For this review, take the finished solid that the model builds, in its own axes (mm). A direction names the side the tool comes from. Give positions to 0.01 mm unless a question says otherwise; leave off trailing zeros. Write each loop counter-clockwise with the first axis right and the second up, starting at its lowest first coordinate (ties: lowest second). Pieces come first, ordered by that corner, then holes. Notation, with made-up numbers: M -16.5,54.5 L -3.5,54.5 A20 ccw -3.5,87.5 Z; hole C 59,0.25 d9. An arc over 180 degrees is marked long. Write item = value, one per line.
```python
from build123d import *

# Parameters (mm, degrees)
SKETCH1_W           = 45
SKETCH1_H           = 6
BOSS_EXTRUDE1_DEPTH = 6


with BuildPart() as part:
    # Sketch1 → Boss-Extrude1 (new body)
    with BuildSketch(Plane.XY):
        Polygon((127.972610893, -160.108528092), (-86.474936563, -160.108528092), (-86.474936563, -401.007755411), (127.972610893, -401.007755411), (157.972610893, -401.007755411), (163.972610893, -401.007755411), (163.972610893, -366.007755411), (157.972610893, -366.007755411), (157.972610893, -340.782948582), (163.972610893, -340.782948582), (163.972610893, -305.782948582), (157.972610893, -305.782948582), (157.972610893, -255.333334922), (163.972610893, -255.333334922), (163.972610893, -220.333334922), (157.972610893, -220.333334922), (157.972610893, -195.108528092), (163.972610893, -195.108528092), (163.972610893, -160.108528092), (157.972610893, -160.108528092), align=None)
        with Locations((-36.751162835, -237.558141752)):
            Rectangle(SKETCH1_W, SKETCH1_H, mode=Mode.SUBTRACT)
        with Locations((78.248837165, -237.558141752)):
            Rectangle(SKETCH1_W, SKETCH1_H, mode=Mode.SUBTRACT)
        with Locations((-36.751162835, -177.558141752)):
            Rectangle(SKETCH1_W, SKETCH1_H, mode=Mode.SUBTRACT)
        with Locations((78.248837165, -177.558141752)):
            Rectangle(SKETCH1_W, SKETCH1_H, mode=Mode.SUBTRACT)
        with Locations((-36.751162835, -383.558141752)):
            Rectangle(SKETCH1_W, SKETCH1_H, mode=Mode.SUBTRACT)
        with Locations((78.248837165, -383.558141752)):
            Rectangle(SKETCH1_W, SKETCH1_H, mode=Mode.SUBTRACT)
        with Locations((78.248837165, -323.558141752)):
            Rectangle(SKETCH1_W, SKETCH1_H, mode=Mode.SUBTRACT)
        with Locations((-36.751162835, -323.558141752)):
            Rectangle(SKETCH1_W, SKETCH1_H, mode=Mode.SUBTRACT)
        with BuildLine():
            Line((54.167727184, -246.324076289), (109.370044405, -246.324076289))
            ThreePointArc((109.370044405, -246.324076289), (116.441112216, -249.253008477), (119.370044405, -256.324076289))
            Line((119.370044405, -256.324076289), (119.370044405, -304.792207215))
            ThreePointArc((119.370044405, -304.792207215), (116.441112216, -311.863275027), (109.370044405, -314.792207215))
            Line((109.370044405, -314.792207215), (54.167727184, -314.792207215))
            ThreePointArc((54.167727184, -314.792207215), (47.096659372, -311.863275027), (44.167727184, -304.792207215))
            Line((44.167727184, -304.792207215), (44.167727184, -256.324076289))
            ThreePointArc((44.167727184, -256.324076289), (47.096659372, -249.253008477), (54.167727184, -246.324076289))
        make_face(mode=Mode.SUBTRACT)
    extrude(amount=BOSS_EXTRUDE1_DEPTH)


solid = part.part
```
1. We need section A-A, the plane x = -49.5. Write out the cut boundary in (y, z), then the cut area to 3 significant figures.
Responses:
outline = M -401.01,0 L -386.56,0 L -386.56,6 L -401.01,6 Z; M -380.56,0 L -326.56,0 L -326.56,6 L -380.56,6 Z; M -320.56,0 L -240.56,0 L -240.56,6 L -320.56,6 Z; M -234.56,0 L -180.56,0 L -180.56,6 L -234.56,6 Z; M -174.56,0 L -160.11,0 L -160.11,6 L -174.56,6 Z
area = 1,300 mm2
2. Machinability: for faces 4 (the face through (-86.475, -279, 3)), 5 (the face through (157.973, -354, 3)), 6 (the face through (-37, -326.558, 3)), which of the approach directions +Z, -Z, +X, -X, +Y, -Y give a long, thin tool a straight path to every point of the face, cutting with its end or side? Answer none if there is none.
Responses:
face_4 = +Z, -Z, -X, +Y, -Y
face_5 = +Z, -Z, +X
face_6 = +Z, -Z
3. We need section C-C, the plane y = -265.5. Write out the cut boundary in (x, z), then the cut area to 3 significant figures.
Responses:
outline = M -86.47,0 L 44.17,0 L 44.17,6 L -86.47,6 Z; M 119.37,0 L 157.97,0 L 157.97,6 L 119.37,6 Z
area = 1,020 mm2
4. We need section B-B, the plane x = 68. Write out the cut boundary in (y, z).
Responses:
outline = M -401.01,0 L -386.56,0 L -386.56,6 L -401.01,6 Z; M -380.56,0 L -326.56,0 L -326.56,6 L -380.56,6 Z; M -320.56,0 L -314.79,0 L -314.79,6 L -320.56,6 Z; M -246.32,0 L -240.56,0 L -240.56,6 L -246.32,6 Z; M -234.56,0 L -180.56,0 L -180.56,6 L -234.56,6 Z; M -174.56,0 L -160.11,0 L -160.11,6 L -174.56,6 Z
5. We need section D-D, the plane z = 3.25. Count the separate pieces of the cut face and the enclosed holes in it, then the cut area to 3 significant figures.
Responses:
separate_pieces = 1
enclosed_holes = 9
area = 52,500 mm2
6. Insertion check: P1, Ø3, axis at y = -213.5, z = 3.5, coming from the +X side. The pin has a flat end and moves straight along its axis. Give the tip position at first contact, or say it passes through.
Responses:
P1 = 157.97
7. For line 1 along Y through (x, z) = (-36.5, 2.7); line 2 along Y through (x, z) = (82.5, 0.6); line 3 along X through (y, z) = (-270, 2.2), list the stretches that pass through material, from the lowest coordinate up. Write a range as from..to.
Responses:
line_1 = -401.01..-386.56, -380.56..-326.56, -320.56..-240.56, -234.56..-180.56, -174.56..-160.11
line_2 = -401.01..-386.56, -380.56..-326.56, -320.56..-314.79, -246.32..-240.56, -234.56..-180.56, -174.56..-160.11
line_3 = -86.47..44.17, 119.37..157.97
8. The part is to be moulded in two halves that separate along Y. For faces 1 (the face through (37, -401.008, 3)), 2 (the face through (55.749, -384, 3)), 3 (the face through (37, -279, 0)), say which applies: +Y half, -Y half, draft (parallel to the pull), parting line (faces both ways), or undercut.
Responses:
face_1 = -Y half
face_2 = undercut
face_3 = draft
